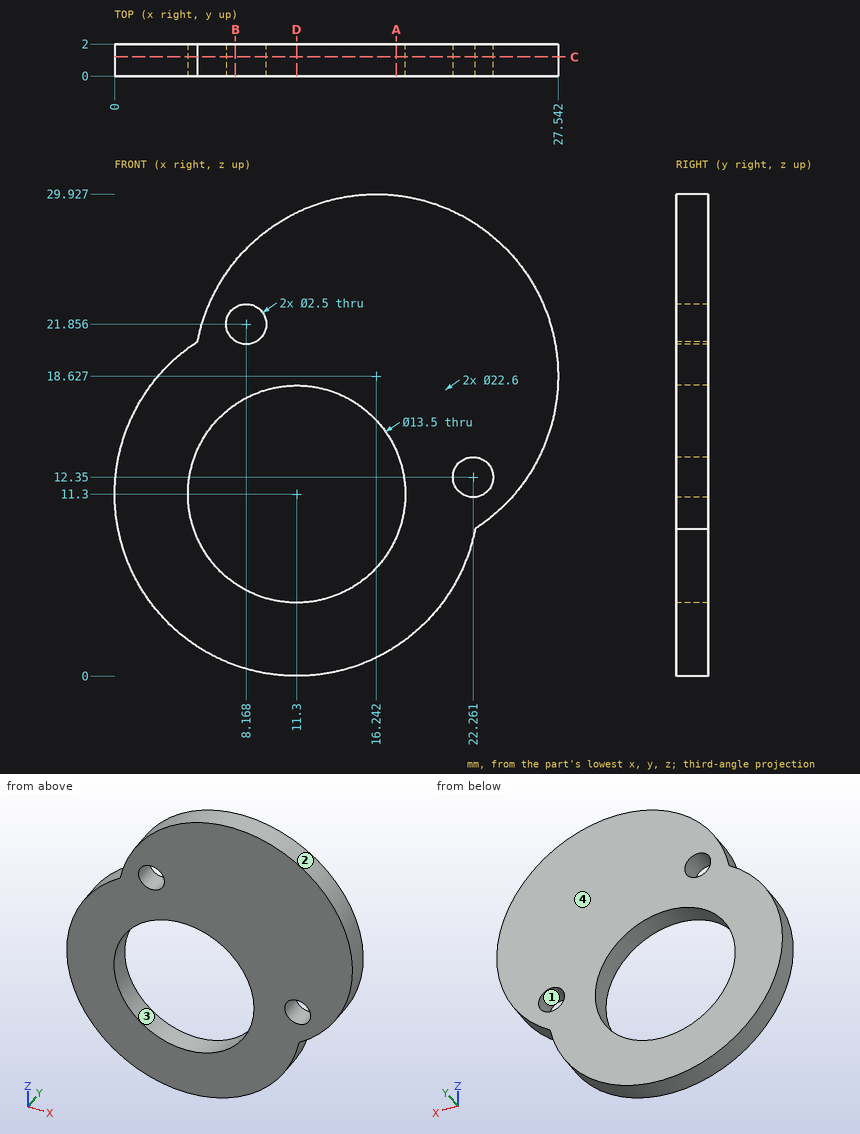
Study the drawing (mm; zero at the part's minimum x, y, z) and answer. Give positions to 0.01 mm unless a question says otherwise; leave off trailing zeros. Write each loop counter-clockwise with the first axis right and the second up, starting at its lowest first coordinate (ties: lowest second). Pieces come first, ordered by that corner, then holes. Notation, with made-up numbers: M -27,12 L 19,12 A26 cw 19,27 Z; hole C 89.5,77 d2. An arc over 180 degrees is marked long. Put each result on its own line as item: value. Start each with the question number.
1. The part is cut by section D-D, the plane x = 11.3. Give the vertices of the cut face in (y, z).
2. For a pull along Z with two mould halves and no side action, classify the marked faces 1, 2, 3 and 4 as released by +Z, released by -Z, zero draft, split by the parting line, or undercut.
3. Each of these flat-tipped pins is pushed along its axis until it touches: pin 1 Ø1 at (y, z) = (0.5, 6.5) entering from +X; pin 2 Ø2 at (x, z) = (22.26, 12.35) entering from -Y. Where does it stop, or does it pass through?
4. The part is cut by section C-C, the plane y = 1.2. Give the vertices of the cut face in (x, z), and give its area (3 significant figures).
5. Consider line 1 along X through (y, z) = (0.75, 12) (1 decimal); line 2 along Z through (x, y) = (9, 1.05) (1 decimal); line 3 along X through (y, z) = (0.35, 22.5) (1 decimal). Determine where each line is inside the solid, lowest interval first.
6. The part is cut by section A-A, the plane x = 17.5. Give the vertices of the cut face in (y, z).
7. The part is cut by section B-B, the plane x = 7.5. Give the vertices of the cut face in (y, z).
Final values:
1. outline: M 0,0 L 2,0 L 2,4.55 L 0,4.55 Z; M 0,18.05 L 2,18.05 L 2,28.79 L 0,28.79 Z
2. face 1: undercut
2. face 2: split by the parting line
2. face 3: undercut
2. face 4: zero draft
3. pin 1: stops at x = 21.75
3. pin 2: passes through
4. outline: M 5.15,20.78 A11.3 ccw long 22.39,9.15 A11.3 ccw long Z; hole C 11.3,11.3 d13.5; hole C 8.17,21.86 d2.5; hole C 22.26,12.35 d2.5
4. area: 443 mm²
5. line 1: x = 0 to 4.6, 18 to 21.1, 23.5 to 25.4
5. line 2: z = 0.2 to 5, 17.6 to 20.9, 22.8 to 27.3
5. line 3: x = 5.6 to 7.1, 9.2 to 26.9
6. outline: M 0,1.85 L 2,1.85 L 2,8.63 L 0,8.63 Z; M 0,13.97 L 2,13.97 L 2,29.86 L 0,29.86 Z
7. outline: M 0,0.66 L 2,0.66 L 2,5.72 L 0,5.72 Z; M 0,16.88 L 2,16.88 L 2,20.8 L 0,20.8 Z; M 0,22.91 L 2,22.91 L 2,25.79 L 0,25.79 Z
